Verification items for the finished model (mm, model axes). Face numbers are marked on the shaded views. A direction names the side the tool comes from. Coordinates: 2 decimals unless noted, no trailing zeros. Order: outer loops, then holes, each group sorted by start corner. A loop starts at its lowest first (then second) coordinate and runs counter-clockwise, first axis right, second up. Notation, with made-up numbers: M 75.25,32 L 131.25,32 A28 cw 131.25,57 Z; hole C 36.25,15 d9. An arc over 180 degrees is marked long. Return JSON: item names as keys, results as strings. Group by question number.
Q1. Section check C-C, the plane z = 23.5. Enter the section's corners in (x, y), then the cut area to 3 significant figures.
Q2. Go/stop test with flat-tipped pins: pin 1 Ø12 at (x, z) = (-7, 14.5) entering from -Y; pin 2 Ø2.5 at (x, y) = (0, -7.5) entering from +Z; pin 3 Ø10 at (x, z) = (8, 7.5) entering from -Y. Record where each tip stops, or that it passes through.
Q3. Section check A-A, the plane y = 0. Enter the section's corners in (x, z), then the cut area to 3 significant figures.
Q4. Mould release check, pull along Y, two halves, no side actions. Record for the marked faces 4, 5 and 6: pulls with the +Y half, pulls with the -Y half, needs draft (parallel to the pull), parting line crosses it, or undercut.
Q5. Thickness scan on probe 1 along Z at (x, y) = (5.5, -6); probe 2 along X at (y, z) = (7.75, 19.25); probe 3 along Z at (x, y) = (0.5, -9.75). Record the ranges inside material, lowest first.
Q6. Section check D-D, the plane y = -3.75. Enter the section's corners in (x, z).
Q7. Access from +Z, -Z, +X, -X, +Y, -Y to the whole of each face (thin tool, end or side, straight path). Record for the marked faces 1, 2 and 3.
Q8. Section check B-B, the plane x = 0. Enter the section's corners in (y, z), then the cut area to 3 significant figures.
from build123d import *
from build123d import SkipClean  # not in build123d's __all__

# Parameters (mm, degrees)
F0_R     = 1.2065
F1_DEPTH = 2.54
F3_DEPTH = 22.86
F4_R     = 2.5
F5_DEPTH = 6.35


# Not quite as in the source:
# - a feature names something its author has since deleted; it is built from what else it names


with BuildPart() as f1:
    # F0 (on Top) → F1 (new body)
    with BuildSketch(Plane.XY):
        with BuildLine():
            ThreePointArc((7.747, -7.9846143326), (2.4553498698, 0), (7.747, 7.9846143326))
            ThreePointArc((7.747, 7.9846143326), (0, 11.1252), (-7.747, 7.9846143326))
            ThreePointArc((-7.747, 7.9846143326), (-2.4553498698, 0), (-7.747, -7.9846143326))
            ThreePointArc((-7.747, -7.9846143326), (0, -11.1252), (7.747, -7.9846143326))
        make_face()
        with BuildLine():
            ThreePointArc((-7.747, -7.9846143326), (-2.4553498698, 0), (-7.747, 7.9846143326))
            ThreePointArc((-7.747, 7.9846143326), (-11.1252, 0), (-7.747, -7.9846143326))
        make_face()
        with Locations((-7.747, 0)):
            Circle(F0_R, mode=Mode.SUBTRACT)
        with BuildLine():
            ThreePointArc((7.747, -7.9846143326), (10.245901606, -4.3349250651), (11.1252, 0))
            ThreePointArc((11.1252, 0), (10.245901606, 4.3349250651), (7.747, 7.9846143326))
            ThreePointArc((7.747, 7.9846143326), (2.4553498698, 0), (7.747, -7.9846143326))
        make_face()
        with Locations((7.747, 0)):
            Circle(F0_R, mode=Mode.SUBTRACT)
    extrude(amount=F1_DEPTH)

    # F2 (on face) → F3 (join)
    with BuildSketch(Plane.XY.offset(2.54)):
        with BuildLine():
            ThreePointArc((-7.747, 7.9846143326), (-2.4553498698, 0), (-7.747, -7.9846143326))
            ThreePointArc((-7.747, -7.9846143326), (0, -11.1252), (7.747, -7.9846143326))
            ThreePointArc((7.747, -7.9846143326), (2.4553498698, 0), (7.747, 7.9846143326))
            ThreePointArc((7.747, 7.9846143326), (0, 11.1252), (-7.747, 7.9846143326))
        make_face()
    with SkipClean():  # cleaning this boolean's faces spoils the solid; the shape is the same uncleaned
        extrude(amount=F3_DEPTH)

    # F4 (on face) → F5 (cut)
    with BuildSketch(Plane.XY.offset(25.4)):
        with Locations((0, 7.62)):
            Circle(F4_R)
        with Locations((0, -7.62)):
            Circle(F4_R)
    extrude(amount=-F5_DEPTH, mode=Mode.SUBTRACT)


solid = f1.part
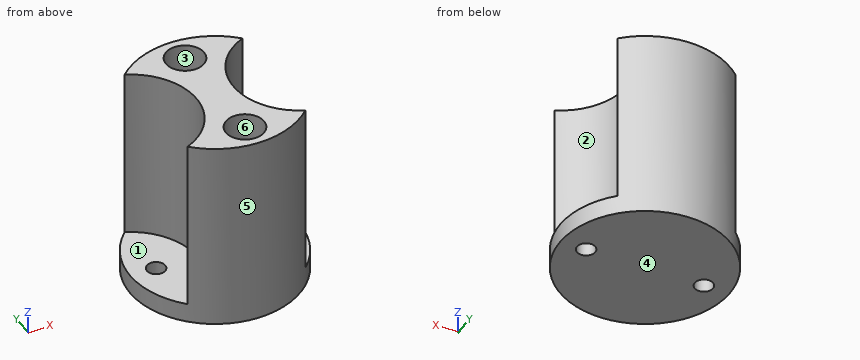
Numbers:
{
 "1": {"outline": "M -7.75,-7.98 A11.13 ccw 7.75,-7.98 A8.67 cw 7.75,7.98 A11.13 ccw -7.75,7.98 A8.67 cw Z; hole C 0,-7.62 d5; hole C 0,7.62 d5", "area": "153 mm2"},
 "2": {"pin 1": "stops at y = -11.08", "pin 2": "stops at z = 19.05", "pin 3": "stops at y = -10.71"},
 "3": {"outline": "M -11.13,0 L -8.95,0 L -8.95,2.54 L -11.13,2.54 Z; M -6.54,0 L 6.54,0 L 6.54,2.54 L 2.46,2.54 L 2.46,25.4 L -2.46,25.4 L -2.46,2.54 L -6.54,2.54 Z; M 8.95,0 L 11.13,0 L 11.13,2.54 L 8.95,2.54 Z", "area": "157 mm2"},
 "4": {"face 4": "needs draft", "face 5": "parting line crosses it", "face 6": "undercut"},
 "5": {"probe 1": "z = 0 to 2.54", "probe 2": "x = -7.24 to -2.5, 2.5 to 7.24", "probe 3": "z = 0 to 19.05"},
 "6": {"outline": "M -10.47,0 L 10.47,0 L 10.47,2.54 L 3.31,2.54 L 3.31,25.4 L -3.31,25.4 L -3.31,2.54 L -10.47,2.54 Z"},
 "7": {"face 1": "+Z, -X", "face 2": "+Z, +X", "face 3": "+Z"},
 "8": {"outline": "M -11.13,0 L 11.13,0 L 11.13,25.4 L 10.12,25.4 L 10.12,19.05 L 5.12,19.05 L 5.12,25.4 L -5.12,25.4 L -5.12,19.05 L -10.12,19.05 L -10.12,25.4 L -11.13,25.4 Z", "area": "502 mm2"}
}
